from build123d import *

# Parameters (mm, degrees)
ESQUISSE1_W             = 80
ESQUISSE1_H             = 169.5
BOSS_EXTRU_1_DEPTH      = 4
ESQUISSE2_R             = 4
ENL_V_MAT_EXTRU_1_DEPTH = 5
ESQUISSE5_R             = 3
ENL_V_MAT_EXTRU_2_DEPTH = 5
ESQUISSE6_W             = 80
ESQUISSE6_H             = 5
BOSS_EXTRU_2_DEPTH      = 6
ESQUISSE7_R             = 2
ENL_V_MAT_EXTRU_5_DEPTH = 11


with BuildPart() as part:
    # Esquisse1 → Boss.-Extru.1 (new body)
    with BuildSketch(Plane.XY):
        with Locations((10.990966959, -33.844488189)):
            Rectangle(ESQUISSE1_W, ESQUISSE1_H)
    extrude(amount=BOSS_EXTRU_1_DEPTH)

    # Esquisse2 → Enlèv. mat.-Extru.1 (cut, through all)
    with BuildSketch(Plane.XY.offset(4)):
        with Locations((-19.009033041, 35.905511811)):
            Circle(ESQUISSE2_R)
        with Locations((40.990966959, 35.905511811)):
            Circle(ESQUISSE2_R)
        with Locations((-19.009033041, -24.094488189)):
            Circle(ESQUISSE2_R)
        with Locations((40.990966959, -24.094488189)):
            Circle(ESQUISSE2_R)
    extrude(amount=-ENL_V_MAT_EXTRU_1_DEPTH, mode=Mode.SUBTRACT)

    # Esquisse5 → Enlèv. mat.-Extru.2 (cut, through all)
    with BuildSketch(Plane.XY.offset(4)):
        with Locations((11.990966959, -108.344488189)):
            Circle(ESQUISSE5_R)
        with Locations((11.990966959, -87.844488189)):
            Circle(ESQUISSE5_R)
    extrude(amount=-ENL_V_MAT_EXTRU_2_DEPTH, mode=Mode.SUBTRACT)

    # Esquisse6 → Boss.-Extru.2 (add)
    with BuildSketch(Plane(origin=(0, 0, 0), x_dir=(-1, 0, 0), z_dir=(0, 0, -1))):
        with Locations((-10.990966959, 48.405511811)):
            Rectangle(ESQUISSE6_W, ESQUISSE6_H)
    extrude(amount=BOSS_EXTRU_2_DEPTH)

    # Esquisse7 → Enlèv. mat.-Extru.5 (cut, through all)
    with BuildSketch(Plane.XY.offset(4)):
        with Locations((7.490966959, -49.894488189)):
            Circle(ESQUISSE7_R)
        with Locations((25.390966959, -27.494488189)):
            Circle(ESQUISSE7_R)
        with Locations((24.590966959, -58.894488189)):
            Circle(ESQUISSE7_R)
    extrude(amount=-ENL_V_MAT_EXTRU_5_DEPTH, mode=Mode.SUBTRACT)


solid = part.part
Geometry: final body of the model. Coordinates: model frame, mm. Give positions to 0.01 mm unless a question says otherwise; leave off trailing zeros. Write each loop counter-clockwise with the first axis right and the second up, starting at its lowest first coordinate (ties: lowest second). Pieces come first, ordered by that corner, then holes.
(1) First-contact query: P1, Ø6.5, axis at x = 7.49, y = -49.89, coming from the +Z side; P2, Ø1.8, axis at x = 3, z = -2, coming from the -Y side; P3, Ø13, axis at x = 40.99, y = -24.09, coming from the -Z side. Flat tips, straight axial feed; report the tip coordinate or a pass-through.
(2) Cut plane B-B, the plane y = 0. Return loops of the section in (x, z).
(3) Cut plane D-D, the plane x = -20. Return loops of the section in (y, z), then the cut area to 3 significant figures.
(4) Cut plane C-C, the plane z = -2.75. Return loops of the section in (x, y), then the cut area to 3 significant figures.
(5) Mould query, pull axis Y, two halves, no side actions, for faces 1 (the cylindrical face through (11.341, -90.773, 2.028)), 2 (the flat face through (12, 45.906, -3)), 3 (the flat face through (10, -35, 0)). Classes: released by +Y, released by -Y, zero draft, split by the parting line, or undercut.
(6) Cut plane A-A, the plane x = 38.5. Return loops of the section in (y, z).
(7) Ray query, line 1 (Y direction, x = 44.5, z = 2.5); line 2 (Z direction, x = 26.5, y = 8); line 3 (Y direction, x = 46.5, z = -1.5). Return the intervals inside material, ascending.
Values follow:
1. P1: stops at z = 4
1. P2: stops at y = 45.91
1. P3: stops at z = 0
2. outline: (-29.01, 0) - (50.99, 0) - (50.99, 4) - (-29.01, 4) - close
3. outline: (-118.59, 0) - (-27.97, 0) - (-27.97, 4) - (-118.59, 4) - close; (-20.22, 0) - (32.03, 0) - (32.03, 4) - (-20.22, 4) - close; (39.78, 0) - (45.91, 0) - (45.91, -6) - (50.91, -6) - (50.91, 4) - (39.78, 4) - close
3. area: 646 mm2
4. outline: (-29.01, 45.91) - (50.99, 45.91) - (50.99, 50.91) - (-29.01, 50.91) - close
4. area: 400 mm2
5. face 1: undercut
5. face 2: released by -Y
5. face 3: zero draft
6. outline: (-118.59, 0) - (-27.22, 0) - (-27.22, 4) - (-118.59, 4) - close; (-20.96, 0) - (32.78, 0) - (32.78, 4) - (-20.96, 4) - close; (39.04, 0) - (45.91, 0) - (45.91, -6) - (50.91, -6) - (50.91, 4) - (39.04, 4) - close
7. line 1: y = -118.59 to -26.01, -22.17 to 33.99, 37.83 to 50.91
7. line 2: z = 0 to 4
7. line 3: y = 45.91 to 50.91
